Design review of the part built by this model. Coordinates are the model's own, in mm. Coordinates: 2 decimals unless noted, no trailing zeros. Write each loop counter-clockwise with the first axis right and the second up, starting at its lowest first coordinate (ties: lowest second). Pieces come first, ordered by that corner, then holes. Notation, with made-up numbers: M 31,-13 L 40,-13 A22 cw 40,25 Z; hole C 28,72.25 d5. An arc over 180 degrees is marked long. Write each question's results on one line, items separated by ' | '. Start each with the question number.
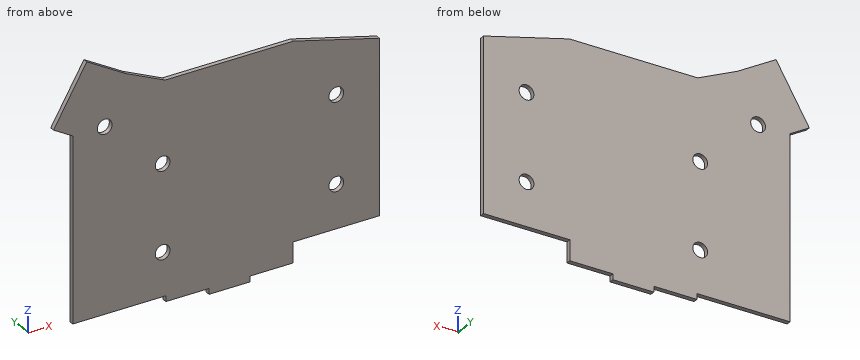
```python
from build123d import *

# Parameters (mm, degrees)
SKETCH_1_R      = 3.25
EXTRUDE_1_DEPTH = 2


with BuildPart() as part:
    # Эскиз1 → Бобышка-Вытянуть1 (new body)
    with BuildSketch(Plane(origin=(0, 0, 0), x_dir=(1, 0, 0), z_dir=(0, 1, 0))):
        Polygon((0, 0), (0, -80.5), (-8.5, -85.5), (6.153232532, -110.410495305), (23.153232532, -100.410495305), (40.653232532, -92.410495305), (97.153232532, -92.410495305), (135, -82.5), (135, -6.5), (97, -6.5), (97, 2.5), (78, 2.5), (78, 5), (60, 5), (60, 2.5), (41, 2.5), (41, 0), align=None)
        with Locations((14.07, -80.258)):
            Circle(SKETCH_1_R, mode=Mode.SUBTRACT)
        with Locations((39.57, -56.958)):
            Circle(SKETCH_1_R, mode=Mode.SUBTRACT)
        with Locations((116.07, -63.958)):
            Circle(SKETCH_1_R, mode=Mode.SUBTRACT)
        with Locations((116.07, -25.658)):
            Circle(SKETCH_1_R, mode=Mode.SUBTRACT)
        with Locations((39.57, -19.048)):
            Circle(SKETCH_1_R, mode=Mode.SUBTRACT)
    extrude(amount=EXTRUDE_1_DEPTH)


solid = part.part
```
Item 1: We need section D-D on x = 94.5. State the section outline as (y, z) points, then the cut area to 3 significant figures.
Item 2: We need section C-C on x = 14.07. State the section outline as (y, z) points.
Item 3: Wall thickness on L1, parallel to Z at x = 116.07, y = 1.25; L2, parallel to X at y = 0.65, z = 63.5; L3, parallel to Z at x = 115.5, y = 1.85: over which ranges is each line inside the solid? List them lowest first.
Item 4: We need section B-B on y = 0.75. State the section outline as (x, z) points, then the cut area to 3 significant figures.
Item 5: We need section A-A on x = 116.07. State the section outline as (y, z) points, then the cut area to 3 significant figures.
Item 6: Insertion check: pin 1 Ø5 at (x, z) = (39.57, 56.958) entering from +Y; pin 2 Ø0.6 at (x, y) = (118, 1) entering from -Z; pin 3 Ø0.6 at (x, y) = (55, 1.5) entering from -Z; pin 4 Ø1 at (x, y) = (60, 2) entering from +Z. Each pin has a flat end and moves straight along its axis. Give the tip position at first contact, or say it passes through.
Answer:
1) outline: M 0,-2.5 L 2,-2.5 L 2,92.41 L 0,92.41 Z | area: 190 mm^2
2) outline: M 0,0 L 2,0 L 2,77.01 L 0,77.01 Z; M 0,83.51 L 2,83.51 L 2,105.75 L 0,105.75 Z
3) L1: z = 6.5 to 22.41, 28.91 to 60.71, 67.21 to 87.46 | L2: x = 0 to 112.85, 119.29 to 135 | L3: z = 6.5 to 22.46, 28.86 to 60.76, 67.16 to 87.61
4) outline: M -8.5,85.5 L 0,80.5 L 0,0 L 41,0 L 41,-2.5 L 60,-2.5 L 60,-5 L 78,-5 L 78,-2.5 L 97,-2.5 L 97,6.5 L 135,6.5 L 135,82.5 L 97.15,92.41 L 40.65,92.41 L 23.15,100.41 L 6.15,110.41 Z; hole C 14.07,80.26 d6.5; hole C 39.57,19.05 d6.5; hole C 39.57,56.96 d6.5; hole C 116.07,25.66 d6.5; hole C 116.07,63.96 d6.5 | area: 12,500 mm^2
5) outline: M 0,6.5 L 2,6.5 L 2,22.41 L 0,22.41 Z; M 0,28.91 L 2,28.91 L 2,60.71 L 0,60.71 Z; M 0,67.21 L 2,67.21 L 2,87.46 L 0,87.46 Z | area: 136 mm^2
6) pin 1: passes through | pin 2: stops at z = 6.5 | pin 3: stops at z = -2.5 | pin 4: stops at z = 92.41
